Input: part model. Units: mm. Frame: model coordinates. Round coordinates to 2 decimals unless told otherwise and drop trailing zeros. Loops run counter-clockwise (first coordinate to the right, second up) from the corner with the lowest first, then second, coordinate; pieces in that order, holes last. Notation, with made-up numbers: (-28.75, -15) -> (22.25, -15) arc R13 ccw to (22.25, 9) -> close; hole circle Ø3 at (-10.5, 69). An arc over 180 degrees is marked (long way). Answer in a Markdown table with one row per item. Add a question column.
Q1. Pin query (flat end, axial travel): pin 1 (2.5 mm diameter, centred on x = -10, y = 6.5, fed in from -Z); pin 2 (4 mm diameter, centred on y = 2.5, z = -85, fed in from -X); pin 3 (5 mm diameter, centred on y = 5.5, z = -152, fed in from -X). Return the tip coordinate at first contact, or that it passes through.
Q2. Section D-D, the plane z = -29. Output: boundary loops of the cut face in (x, y), and give its area (3 significant figures).
Q3. Section C-C, the plane x = 16. Output: boundary loops of the cut face in (y, z).
Q4. Section B-B, the plane y = 8.5. Output: boundary loops of the cut face in (x, z), and give its area (3 significant figures).
Q5. Section A-A, the plane z = 0. Output: boundary loops of the cut face in (x, y) (3 decimals).
Q6. Ray query, L1, parallel to X at y = 3.05, z = 0 (3 decimals); L2, parallel to Y at x = -10.5, z = -67.5; L3, parallel to Z at x = -12, y = 6.25. Return the intervals inside material, ascending. Write a range as from..to.
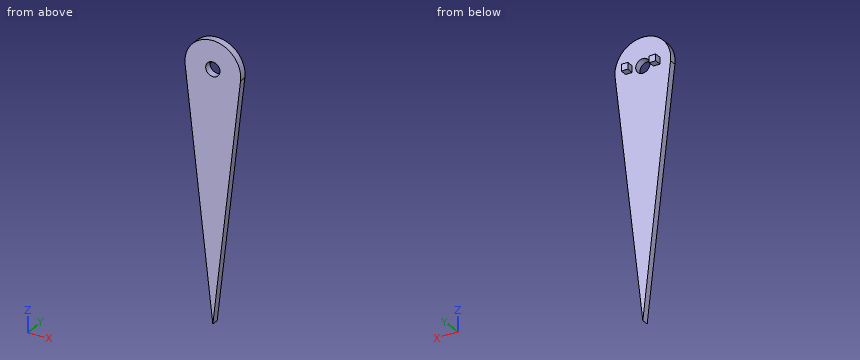
```python
from build123d import *

# Parameters (mm, degrees)
SKETCH1_R           = 5.125
BOSS_EXTRUDE1_DEPTH = 5
SKETCH2_W           = 4.7
SKETCH2_H           = 4.7
BOSS_EXTRUDE2_DEPTH = 5


with BuildPart() as part:
    # Sketch1 → Boss-Extrude1 (new body)
    with BuildSketch(Plane(origin=(0, 0, 0), x_dir=(1, 0, 0), z_dir=(0, 1, 0))):
        with BuildLine():
            Line((-19.872284397, 2.256615355), (0, 177.256615355))
            Line((0, 177.256615355), (19.872284397, 2.256615355))
            ThreePointArc((19.872284397, 2.256615355), (0, -20), (-19.872284397, 2.256615355))
        make_face()
        Circle(SKETCH1_R, mode=Mode.SUBTRACT)
    extrude(amount=BOSS_EXTRUDE1_DEPTH)

    # Sketch2 → Boss-Extrude2 (add)
    with BuildSketch(Plane(origin=(0, 5, 0), x_dir=(1, 0, 0), z_dir=(0, 1, 0))):
        with Locations((10, 0)):
            Rectangle(SKETCH2_W, SKETCH2_H)
        with Locations((-10, 0)):
            Rectangle(SKETCH2_W, SKETCH2_H)
    extrude(amount=BOSS_EXTRUDE2_DEPTH)


solid = part.part
```
Answer block:
| question | item | result |
|---|---|---|
| 1 | pin 1 | z = -2.35 |
| 1 | pin 2 | x = -10.7 |
| 1 | pin 3 | x = -3.15 |
| 2 | outline | (-16.84, 0) -> (16.84, 0) -> (16.84, 5) -> (-16.84, 5) -> close |
| 2 | area | 168 mm^2 |
| 3 | outline | (0, -36.36) -> (5, -36.36) -> (5, 12) -> (0, 12) -> close |
| 4 | outline | (-12.35, -2.35) -> (-7.65, -2.35) -> (-7.65, 2.35) -> (-12.35, 2.35) -> close; (7.65, -2.35) -> (12.35, -2.35) -> (12.35, 2.35) -> (7.65, 2.35) -> close |
| 4 | area | 44.2 mm^2 |
| 5 | outline | (-20, 0) -> (-5.125, 0) -> (-5.125, 5) -> (-7.65, 5) -> (-7.65, 10) -> (-12.35, 10) -> (-12.35, 5) -> (-20, 5) -> close; (5.125, 0) -> (20, 0) -> (20, 5) -> (12.35, 5) -> (12.35, 10) -> (7.65, 10) -> (7.65, 5) -> (5.125, 5) -> close |
| 6 | L1 | -20..-5.125, 5.125..20 |
| 6 | L2 | 0..5 |
| 6 | L3 | -2.35..2.35 |
